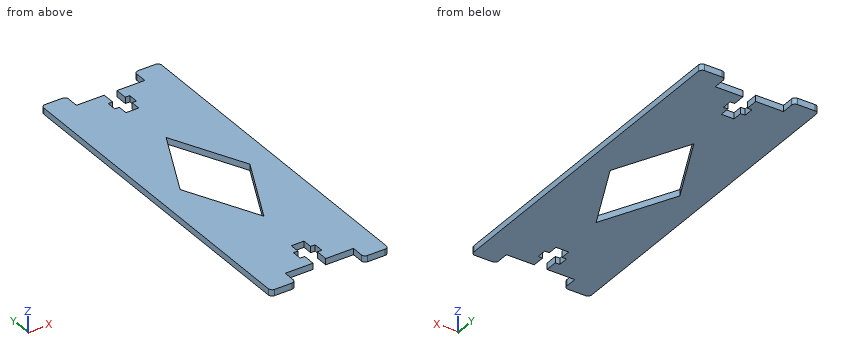
```python
from build123d import *

# Parameters (mm, degrees)
EXTRUDE_1_DEPTH = 2
FILLET_1_R      = 1.2


with BuildPart() as part:
    # 草图1 → 凸台-拉伸1 (new body)
    with BuildSketch(Plane.XY):
        Polygon((15.059090909, 15.4), (15.059090909, -94.6), (7.059090909, -94.6), (7.059090909, -89.6), (-1.890909091, -89.6), (-1.890909091, -85.6), (-0.440909091, -85.6), (-0.440909091, -82.4), (-1.890909091, -82.4), (-1.890909091, -79.2), (-5.990909091, -79.2), (-5.990909091, -82.4), (-7.440909091, -82.4), (-7.440909091, -85.6), (-5.990909091, -85.6), (-5.990909091, -89.6), (-14.940909091, -89.6), (-14.940909091, -94.6), (-22.940909091, -94.6), (-22.940909091, 15.4), (-14.940909091, 15.4), (-14.940909091, 10.4), (-5.990909091, 10.4), (-5.990909091, 6.4), (-7.440909091, 6.4), (-7.440909091, 3.2), (-5.990909091, 3.2), (-5.990909091, 0), (-1.890909091, 0), (-1.890909091, 3.2), (-0.440909091, 3.2), (-0.440909091, 6.4), (-1.890909091, 6.4), (-1.890909091, 10.4), (7.059090909, 10.4), (7.059090909, 15.4), align=None)
        Polygon((-3.940909091, -16.181864614), (-15.17688314, -39.6), (-3.940909091, -63.018135386), (7.295064958, -39.6), align=None, mode=Mode.SUBTRACT)
    extrude(amount=EXTRUDE_1_DEPTH)

    # 圆角1
    fillet_1_edges = [part.edges().sort_by_distance(p)[0] for p in [
        (7.059090909, 15.4, 1),
        (15.059090909, 15.4, 1),
        (15.059090909, -94.6, 1),
        (7.059090909, -94.6, 1),
        (-14.940909091, -94.6, 1),
        (-22.940909091, -94.6, 1),
        (-22.940909091, 15.4, 1),
        (-14.940909091, 15.4, 1),
    ]]
    fillet(fillet_1_edges, radius=FILLET_1_R)


solid = part.part
```
Model file for the job. Use its own axes, mm. Round coordinates to 2 decimals unless told otherwise and drop trailing zeros. Order: outer loops, then holes, each group sorted by start corner. A loop starts at its lowest first (then second) coordinate and runs counter-clockwise, first axis right, second up. Notation, with made-up numbers: (-35.5, 54.5) -> (-9.5, 54.5) arc R29 ccw to (-9.5, 76.5) -> close; hole circle Ø7 at (8.25, 33). An arc over 180 degrees is marked (long way). Use one line per item in the form item = value.
Item 1: Drill centre lines: line 1 (X direction, y = -82.5, z = 0.4); line 2 (X direction, y = -80, z = 1.8); line 3 (Y direction, x = -7, z = 0.35). Where is each one in solid material? Low to high.
Returned:
line_1 = -22.94 to -7.44, -0.44 to 15.06
line_2 = -22.94 to -5.99, -1.89 to 15.06
line_3 = -89.6 to -85.6, -82.4 to -56.64, -22.56 to 3.2, 6.4 to 10.4
Item 2: Flat gauge pins, fed straight in: pin 1 Ø0.7 at (x, z) = (-6.5, 1.5) entering from -Y; pin 2 Ø0.7 at (x, z) = (-7, 1) entering from +Y. Where does each tip first touch, or does it go through?
Returned:
pin_1 = -89.6
pin_2 = 10.4
Item 3: Cut at A-A, the plane y = -50.5. Write the cut outline in (x, z), and give its area (3 significant figures).
Returned:
outline = (-22.94, 0) -> (-9.95, 0) -> (-9.95, 2) -> (-22.94, 2) -> close; (2.07, 0) -> (15.06, 0) -> (15.06, 2) -> (2.07, 2) -> close
area = 52.0 mm^2
Item 4: Cut at B-B, the plane x = -9. Write the cut outline in (y, z).
Returned:
outline = (-89.6, 0) -> (-52.47, 0) -> (-52.47, 2) -> (-89.6, 2) -> close; (-26.73, 0) -> (10.4, 0) -> (10.4, 2) -> (-26.73, 2) -> close
